Verification items for the finished model (mm, model axes). A direction names the side the tool comes from. Give positions to 0.01 mm unless a question says otherwise; leave off trailing zeros. Order: outer loops, then holes, each group sorted by start corner. A loop starts at its lowest first (then second) coordinate and runs counter-clockwise, first axis right, second up. Notation, with made-up numbers: (30.5, 69) -> (73.5, 69) arc R16 cw to (73.5, 87) -> close; hole circle Ø7 at (79, 51). An arc over 180 degrees is marked (long way). Return JSON: item names as keys, results as strings. Group by question number.
(1) Tool access check on faces 1 (the face through (20.574, 31, -36)), 2 (the face through (43, 32.766, -33)), 3 (the face through (29, 16.002, -25)), 4 (the face through (43, 28.702, -33)), 5 (the face through (7.874, 31, -36)). Record the directions out of +Z, -Z, +X, -X, +Y, -Y that give a thin tool (end or side, any length) a straight path to the whole face; none if there is none.
(2) Cross-section at A-A on z = -38.1. Enter the section's corners in (x, y), then the cut area to 3 significant figures.
(3) Release check for a two-part mould opening along Z. For faces 6 (the face through (49.276, 31, -36)), 7 (the face through (28, 20, -28.702)), 8 (the face through (40.7, 30.8, -34.7)) record: pulls with the +Z half, pulls with the -Z half, needs draft (parallel to the pull), parting line crosses it, or undercut.
(4) Thickness scan on line 1 along X through (y, z) = (12, -3); line 2 along X through (y, z) = (31, -32); line 3 along Z through (x, y) = (7, 34). Record the ranges inside material, lowest first.
(5) Depth check by flat-ended pin: pin 1 Ø10 at (x, z) = (13, -39.5) entering from +Y; pin 2 Ø2 at (y, z) = (30, -32.5) entering from +X; pin 3 Ø2 at (x, z) = (28, -25) entering from +Y. Enter the tip coordinate at first touch or a pass-through.
(6) Cross-section at B-B on z = -29.5. Enter the section's corners in (x, y).
(7) Cross-section at D-D on y = 19.5. Enter the section's corners in (x, z) (3 decimals).
(8) Cross-section at C-C on x = 14.5. Enter the section's corners in (y, z), then the cut area to 3 significant figures.
from build123d import *

# Parameters (mm, degrees)
SKETCH1_W          = 57.15
SKETCH1_H          = 28.702
EXTRUDE1_DEPTH     = 41.402
SKETCH2_R          = 2.5527
CUT_EXTRUDE1_DEPTH = 42.402
SKETCH3_R          = 2.0193
CUT_EXTRUDE2_DEPTH = 25.4
SKETCH8_R          = 2.794
CUT_EXTRUDE3_DEPTH = 29.702
SKETCH9_W          = 12.7
SKETCH9_H          = 4.064
EXTRUDE2_DEPTH     = 14.732
SKETCH10_R         = 4.064
CUT_EXTRUDE4_DEPTH = 33.766


with BuildPart() as part:
    # Sketch1 → Extrude1 (new body)
    with BuildSketch(Plane(origin=(0, 0, 0), x_dir=(1, 0, 0), z_dir=(0, 1, 0))):
        with Locations((28.575, 14.351)):
            Rectangle(SKETCH1_W, SKETCH1_H)
    extrude(amount=EXTRUDE1_DEPTH)

    # Sketch2 → Cut-Extrude1 (cut, through all)
    with BuildSketch(Plane(origin=(0, 41.402, 0), x_dir=(-1, 0, 0), z_dir=(0, 1, 0))):
        with Locations((-28.575, -14.351)):
            Circle(SKETCH2_R)
    extrude(amount=-CUT_EXTRUDE1_DEPTH, mode=Mode.SUBTRACT)

    # Sketch3 → Cut-Extrude2 (cut)
    with BuildSketch(Plane(origin=(0, 41.402, 0), x_dir=(-1, 0, 0), z_dir=(0, 1, 0))):
        with Locations((-28.575, -24.638)):
            Circle(SKETCH3_R)
        with Locations((-28.575, -4.064)):
            Circle(SKETCH3_R)
    extrude(amount=-CUT_EXTRUDE2_DEPTH, mode=Mode.SUBTRACT)

    # Sketch8 → Cut-Extrude3 (cut, through all)
    with BuildSketch(Plane(origin=(0, 0, -28.702), x_dir=(-1, 0, 0), z_dir=(0, 0, -1))):
        with Locations((-42.926, 9.652)):
            Circle(SKETCH8_R)
        with Locations((-14.224, 9.652)):
            Circle(SKETCH8_R)
    extrude(amount=-CUT_EXTRUDE3_DEPTH, mode=Mode.SUBTRACT)

    # Sketch9 → Extrude2 (add)
    with BuildSketch(Plane(origin=(0, 0, -28.702), x_dir=(-1, 0, 0), z_dir=(0, 0, -1))):
        with Locations((-42.926, 30.734)):
            Rectangle(SKETCH9_W, SKETCH9_H)
        with Locations((-14.224, 30.734)):
            Rectangle(SKETCH9_W, SKETCH9_H)
    extrude(amount=EXTRUDE2_DEPTH)

    # Sketch10 → Cut-Extrude4 (cut, through all)
    with BuildSketch(Plane(origin=(0, 32.766, 0), x_dir=(-1, 0, 0), z_dir=(0, 1, 0))):
        with Locations((-42.926, -38.1)):
            Circle(SKETCH10_R)
        with Locations((-14.224, -38.1)):
            Circle(SKETCH10_R)
    extrude(amount=-CUT_EXTRUDE4_DEPTH, mode=Mode.SUBTRACT)


solid = part.part
Verdict:
{
 "1": {"face 1": "-Z, +Y, -Y", "face 2": "-Z, +X, -X, +Y", "face 3": "+Y", "face 4": "-Z, +X, -X, -Y", "face 5": "-Z, -X, +Y, -Y"},
 "2": {"outline": "(7.87, 28.7) -> (10.16, 28.7) -> (10.16, 32.77) -> (7.87, 32.77) -> close; (18.29, 28.7) -> (20.57, 28.7) -> (20.57, 32.77) -> (18.29, 32.77) -> close; (36.58, 28.7) -> (38.86, 28.7) -> (38.86, 32.77) -> (36.58, 32.77) -> close; (46.99, 28.7) -> (49.28, 28.7) -> (49.28, 32.77) -> (46.99, 32.77) -> close", "area": "37.2 mm²"},
 "3": {"face 6": "needs draft", "face 7": "pulls with the -Z half", "face 8": "undercut"},
 "4": {"line 1": "0 to 12.71, 15.74 to 41.41, 44.44 to 57.15", "line 2": "7.87 to 20.57, 36.58 to 49.28", "line 3": "-28.7 to 0"},
 "5": {"pin 1": "y = 32.77", "pin 2": "x = 49.28", "pin 3": "y = 16"},
 "6": {"outline": "(7.87, 28.7) -> (20.57, 28.7) -> (20.57, 32.77) -> (7.87, 32.77) -> close; (36.58, 28.7) -> (49.28, 28.7) -> (49.28, 32.77) -> (36.58, 32.77) -> close"},
 "7": {"outline": "(0, -28.702) -> (57.15, -28.702) -> (57.15, 0) -> (0, 0) -> close; hole circle Ø5.105 at (28.575, -14.351); hole circle Ø4.039 at (28.575, -24.638); hole circle Ø4.039 at (28.575, -4.064)"},
 "8": {"outline": "(0, -28.7) -> (6.87, -28.7) -> (6.87, 0) -> (0, 0) -> close; (12.43, -28.7) -> (28.7, -28.7) -> (28.7, -34.05) -> (32.77, -34.05) -> (32.77, -28.7) -> (41.4, -28.7) -> (41.4, 0) -> (12.43, 0) -> close; (28.7, -43.43) -> (32.77, -43.43) -> (32.77, -42.15) -> (28.7, -42.15) -> close", "area": "1,060 mm²"}
}
